Study the drawing (mm; zero at the part's minimum x, y, z) and answer. Round coordinates to 2 decimals unless told otherwise and drop trailing zeros. Loops run counter-clockwise (first coordinate to the right, second up) from the corner with the lowest first, then second, coordinate; pieces in that order, holes last. Notation, with made-up numbers: (-40, 76.25) -> (12, 76.25) arc R9 cw to (12, 80.25) -> close; hole circle Ø4 at (60, 40). An arc over 180 degrees is marked (long way). Answer in a Markdown table with one row per item. Add a question column.
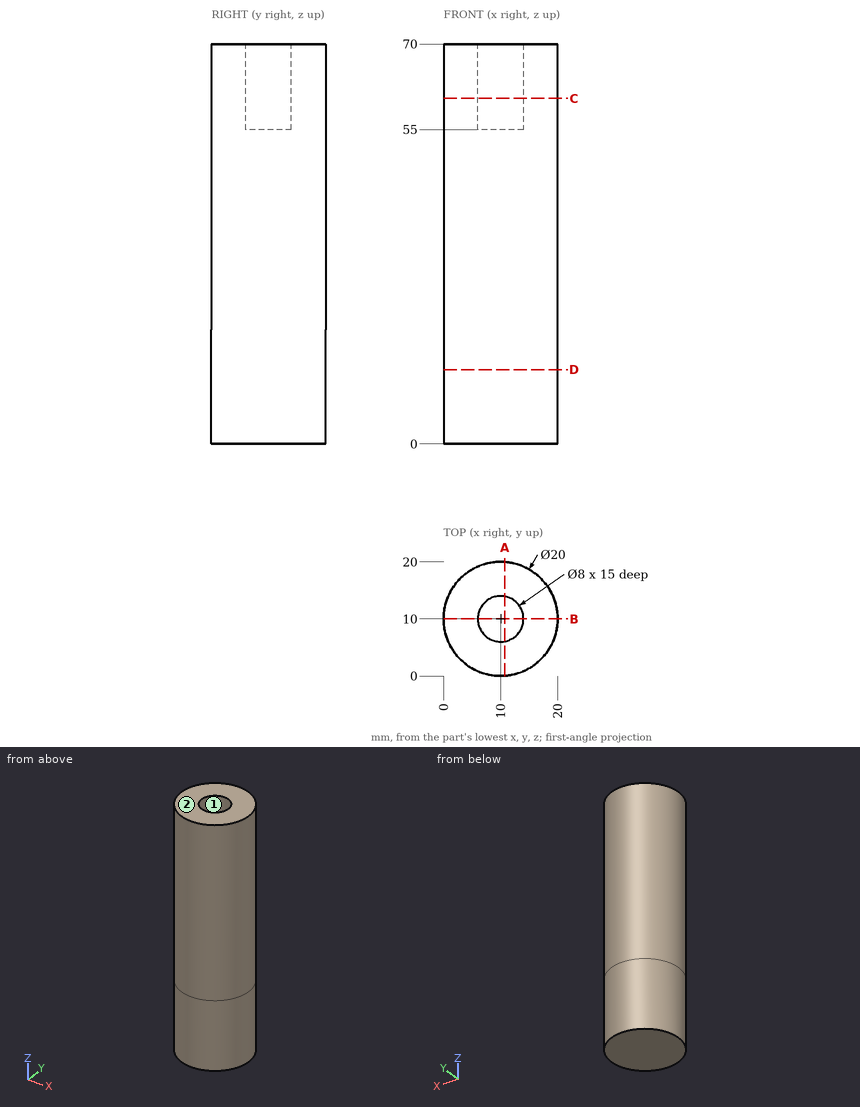
Item 1: Section B-B, the plane y = 10 is taken. Write down the section's boundary in (x, z), and give its area (3 significant figures).
Item 2: Flat-ended cylindrical pins translate along their axes: P1, Ø4, axis at x = 11, y = 11.5, coming from the +Z side; P2, Ø3, axis at y = 12, z = 58.5, coming from the +X side; P3, Ø3, axis at x = 6.5, z = 54.5, coming from the -Y side. Find the tip coordinate at first contact, or state that the pin passes through.
Item 3: Consider L1, parallel to Y at x = 10, z = 58.5; L2, parallel to X at y = 7, z = 62; L3, parallel to Y at x = 10.5, z = 33. Determine where each line is inside the solid, lowest interval first. Write a range as from..to.
Item 4: The mould has two halves that part along X. Classify the marked faces 1 and 2: +X half, -X half, draft (parallel to the pull), parting line (faces both ways), or undercut.
Item 5: Section A-A, the plane x = 10.75 is taken. Write down the section's boundary in (y, z).
Item 6: Section C-C, the plane z = 60.5 is taken. Write down the section's boundary in (x, y), and give its area (3 significant figures).
Item 7: Section D-D, the plane z = 13 is taken. Write down the section's boundary in (x, y).
Here are the results:
| question | item | result |
|---|---|---|
| 1 | outline | (0, 0) -> (20, 0) -> (20, 70) -> (14, 70) -> (14, 55) -> (6, 55) -> (6, 70) -> (0, 70) -> close |
| 1 | area | 1,280 mm² |
| 2 | P1 | stops at z = 55 |
| 2 | P2 | stops at x = 19.99 |
| 2 | P3 | stops at y = 0.2 |
| 3 | L1 | y = 0..6, 14..20 |
| 3 | L2 | x = 0.46..7.35, 12.65..19.54 |
| 3 | L3 | y = 0.01..19.99 |
| 4 | face 1 | undercut |
| 4 | face 2 | draft |
| 5 | outline | (0.03, 0) -> (19.97, 0) -> (19.97, 70) -> (13.93, 70) -> (13.93, 55) -> (6.07, 55) -> (6.07, 70) -> (0.03, 70) -> close |
| 6 | outline | circle Ø20 at (10, 10); hole circle Ø8 at (10, 10) |
| 6 | area | 264 mm² |
| 7 | outline | circle Ø20 at (10, 10) |
